Source: CAD feature listing. Evaluate the final solid. Frame: model axes, mm. A direction names the side the tool comes from. Coordinates: 2 decimals unless noted, no trailing zeros. Write each loop counter-clockwise with the first axis right and the second up, starting at its lowest first coordinate (ties: lowest second). Pieces come first, ordered by that corner, then holes. Notation, with made-up numbers: (-12.5, 35.25) -> (18.5, 35.25) arc R34 ccw to (18.5, 72.25) -> close; hole circle Ø1 at (19, 27). An arc over 180 degrees is marked (long way). Write item = value, one per line.
from build123d import *

# Parameters (mm, degrees)
ESQUISSE1_R             = 3.5
BOSS_EXTRU_1_DEPTH      = 4
ESQUISSE2_R             = 2
ENL_V_MAT_EXTRU_1_DEPTH = 2
BOSS_EXTRU_2_DEPTH      = 2
ESQUISSE4_R             = 1.5
BOSS_EXTRU_3_DEPTH      = 2
ESQUISSE5_R             = 1.5
ENL_V_MAT_EXTRU_2_DEPTH = 2


with BuildPart() as part:
    # Esquisse1 → Boss.-Extru.1 (new body)
    with BuildSketch(Plane(origin=(0, 0, 0), x_dir=(1, 0, 0), z_dir=(0, 1, 0))):
        Circle(ESQUISSE1_R)
    extrude(amount=BOSS_EXTRU_1_DEPTH)

    # Esquisse2 → Enlèv. mat.-Extru.1 (cut)
    with BuildSketch(Plane(origin=(0, 4, 0), x_dir=(1, 0, 0), z_dir=(0, 1, 0))):
        Circle(ESQUISSE2_R)
    extrude(amount=-ENL_V_MAT_EXTRU_1_DEPTH, mode=Mode.SUBTRACT)

    # Esquisse3 → Boss.-Extru.2 (add)
    with BuildSketch(Plane(origin=(0, 0, 0), x_dir=(1, 0, 0), z_dir=(0, 1, 0))):
        Polygon((0, 3.5), (15, 1.5), (15, -1.5), (0, -3.5), align=None)
    boss_extru_2 = extrude(amount=BOSS_EXTRU_2_DEPTH)

    # Esquisse4 → Boss.-Extru.3 (add)
    with BuildSketch(Plane(origin=(0, 2, 0), x_dir=(1, 0, 0), z_dir=(0, 1, 0))):
        with Locations((15, 0)):
            Circle(ESQUISSE4_R)
    boss_extru_3 = extrude(amount=-BOSS_EXTRU_3_DEPTH)

    # Symétrie1: Boss.-Extru.2, Boss.-Extru.3 across plane
    add(boss_extru_2.mirror(Plane(origin=(0, 0, 0), x_dir=(0, 0, 1), z_dir=(1, 0, 0))))
    add(boss_extru_3.mirror(Plane(origin=(0, 0, 0), x_dir=(0, 0, 1), z_dir=(1, 0, 0))))

    # Esquisse5 → Enlèv. mat.-Extru.2 (cut)
    with BuildSketch(Plane(origin=(0, 2, 0), x_dir=(1, 0, 0), z_dir=(0, 1, 0))):
        with Locations((-8.5, 0)):
            Circle(ESQUISSE5_R)
        with Locations((8.5, 0)):
            Circle(ESQUISSE5_R)
    extrude(amount=-ENL_V_MAT_EXTRU_2_DEPTH, mode=Mode.SUBTRACT)


solid = part.part
1) Cut plane C-C, the plane y = 0.35. Output: boundary loops of the cut face in (x, z).
Answer block:
outline = (-15, -1.5) -> (-0.92, -3.38) arc R3.5 ccw to (0.92, -3.38) -> (15, -1.5) arc R1.5 ccw to (15, 1.5) -> (0.92, 3.38) arc R3.5 ccw to (-0.92, 3.38) -> (-15, 1.5) arc R1.5 ccw to start; hole circle Ø3 at (-8.5, 0); hole circle Ø3 at (8.5, 0)
2) Cut plane A-A, the plane z = 0. Output: boundary loops of the cut face in (x, y), and give its area (3 significant figures).
Answer block:
outline = (-16.5, 0) -> (-10, 0) -> (-10, 2) -> (-16.5, 2) -> close; (-7, 0) -> (7, 0) -> (7, 2) -> (3.5, 2) -> (3.5, 4) -> (2, 4) -> (2, 2) -> (-2, 2) -> (-2, 4) -> (-3.5, 4) -> (-3.5, 2) -> (-7, 2) -> close; (10, 0) -> (16.5, 0) -> (16.5, 2) -> (10, 2) -> close
area = 60.0 mm2
3) Cut plane B-B, the plane x = 0. Output: boundary loops of the cut face in (y, z).
Answer block:
outline = (0, -3.5) -> (4, -3.5) -> (4, -2) -> (2, -2) -> (2, 2) -> (4, 2) -> (4, 3.5) -> (0, 3.5) -> close
4) Cut plane D-D, the plane x = -8.5. Output: boundary loops of the cut face in (y, z), and give its area (3 significant figures).
Answer block:
outline = (0, -2.37) -> (2, -2.37) -> (2, -1.5) -> (0, -1.5) -> close; (0, 1.5) -> (2, 1.5) -> (2, 2.37) -> (0, 2.37) -> close
area = 3.47 mm2
5) First-contact query: pin 1 Ø2.5 at (x, z) = (8.5, 0) entering from -Y; pin 2 Ø3 at (x, z) = (13, -2.5) entering from +Y. Flat tips, straight axial feed; report the tip coordinate or a pass-through.
Answer block:
pin_1 = through
pin_2 = 2
6) Reachability of faces 1 (the flat face through (0, 2, 0)), 2 (the flat face through (7.86, 0.99, -2.45)) from +Z, -Z, +X, -X, +Y, -Y: full face, straight path, thin tool, end or side. Return the list, or none.
Answer block:
face_1 = +Y
face_2 = -Z, +X, +Y, -Y
7) Material intervals for probe 1 along X at (y, z) = (0.7, 0); probe 2 along X at (y, z) = (3.1, 0); probe 3 along X at (y, z) = (0.35, -0.5), sorted ascending. Write a range as [from, to].
Answer block:
probe_1 = [-16.5, -10], [-7, 7], [10, 16.5]
probe_2 = [-3.5, -2], [2, 3.5]
probe_3 = [-16.41, -9.91], [-7.09, 7.09], [9.91, 16.41]
